Print and shaded views of the part. All mm, measured from the part's lowest x, y and z. Round coordinates to 2 decimals unless told otherwise and drop trailing zeros. Write each loop counter-clockwise with the first axis right and the second up, starting at its lowest first coordinate (ties: lowest second). Pieces come first, ordered by that corner, then holes. Notation, with made-up numbers: M 78,-7.75 L 90,-7.75 A30 cw 90,24.25 Z; hole C 66,16.5 d4. An arc over 180 degrees is marked long. Write item = value, one per line.
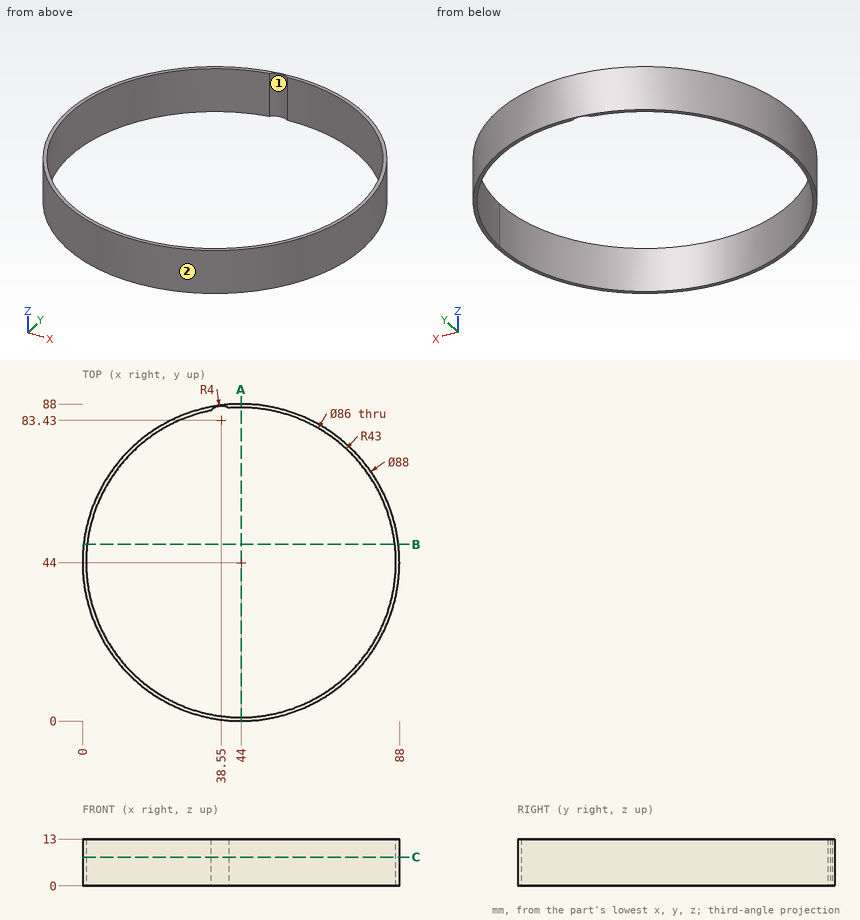
1. Mould opens along X. For the marked faces 1 and 2 say: pulls with the +X half, pulls with the -X half, needs draft (parallel to the pull), parting line crosses it, or undercut.
Responses:
face_1 = undercut
face_2 = parting line crosses it
2. Band-saw the part on B-B (y = 49). List the corners of the cut face in (x, z), plus the area to 3 significant figures.
Responses:
outline = M 0.29,0 L 1.29,0 L 1.29,13 L 0.29,13 Z; M 86.71,0 L 87.71,0 L 87.71,13 L 86.71,13 Z
area = 26.2 mm²
3. Probe probe 1 along Y at (x, z) = (44, 7); probe 2 along Y at (x, z) = (39, 4.25); probe 3 along X at (y, z) = (15, 12.25). List the from-to ranges inside material, lowest first.
Responses:
probe_1 = 0 to 1, 87 to 88
probe_2 = 0.29 to 1.29, 87.4 to 87.71
probe_3 = 10.91 to 12.25, 75.75 to 77.09
4. Flat gauge pins, fed straight in: pin 1 (1 mm diameter, centred on y = 56, z = 6, fed in from +X); pin 2 (1.5 mm diameter, centred on y = 77, z = 11, fed in from -X); pin 3 (2 mm diameter, centred on y = 66.5, z = 11.5, fed in from -X). Where does each tip first touch, or does it go through?
Responses:
pin_1 = 86.47
pin_2 = 14.07
pin_3 = 5.61
5. Band-saw the part on A-A (x = 44). List the corners of the cut face in (y, z).
Responses:
outline = M 0,0 L 1,0 L 1,13 L 0,13 Z; M 87,0 L 88,0 L 88,13 L 87,13 Z
6. Band-saw the part on C-C (z = 8). List the corners of the cut face in (x, y), plus the area to 3 significant figures.
Responses:
outline = C 44,44 d88; hole M 35.65,86.18 A43 ccw long 40.6,86.87 A4 ccw Z
area = 271 mm²
